Can you work these out from the model? Positions are in its coordinate system, mm. A direction names the side the tool comes from. Coordinates: 2 decimals unless noted, no trailing zeros. Loops run counter-clockwise (first coordinate to the right, second up) from the corner with the lowest first, then second, coordinate; pieces in that order, holes last.
```python
from build123d import *

# Parameters (mm, degrees)
SKETCH1_W           = 34.0614
SKETCH1_H           = 60
BOSS_EXTRUDE1_DEPTH = 8.9916
SKETCH2_W           = 34.0614
SKETCH2_H           = 8.9916
BOSS_EXTRUDE2_DEPTH = 51.0084
CUT_EXTRUDE2_REACH  = 10.992
SKETCH5_R           = 2.7686
SKETCH5_R_2         = 2.6416
CUT_EXTRUDE3_REACH  = 62
SKETCH6_R           = 2.7686
BOSS_EXTRUDE3_DEPTH = 34.0614
FILLET1_R           = 4.4958


with BuildPart() as part:
    # Sketch1 → Boss-Extrude1 (new body)
    with BuildSketch(Plane(origin=(0, 0, 0), x_dir=(0, 0, -1), z_dir=(1, 0, 0))):
        Rectangle(SKETCH1_W, SKETCH1_H)
    extrude(amount=BOSS_EXTRUDE1_DEPTH)

    # Sketch2 → Boss-Extrude2 (add)
    with BuildSketch(Plane(origin=(8.9916, 0, 0), x_dir=(0, 0, -1), z_dir=(1, 0, 0))):
        with Locations((0, 25.5042)):
            Rectangle(SKETCH2_W, SKETCH2_H)
    extrude(amount=BOSS_EXTRUDE2_DEPTH)

    # Sketch5 → Cut-Extrude2 (cut, up to next)
    with BuildSketch(Plane(origin=(8.9916, 0, 0), x_dir=(0, 0, -1), z_dir=(1, 0, 0)), mode=Mode.PRIVATE) as cut_extrude2_sk1:
        with Locations((-10.0076, -4.4958)):
            Circle(SKETCH5_R)
    cut_extrude2_tool1 = extrude(cut_extrude2_sk1.sketch, amount=-CUT_EXTRUDE2_REACH, mode=Mode.PRIVATE) & part.part
    add(cut_extrude2_tool1.solids().sort_by_distance((8.9916, -4.4958, 10.0076))[0], mode=Mode.SUBTRACT)
    # Sketch5 → Cut-Extrude2 (cut, up to next)
    with BuildSketch(Plane(origin=(8.9916, 0, 0), x_dir=(0, 0, -1), z_dir=(1, 0, 0)), mode=Mode.PRIVATE) as cut_extrude2_sk2:
        with Locations((10.0076, -4.4958)):
            Circle(SKETCH5_R_2)
    cut_extrude2_tool2 = extrude(cut_extrude2_sk2.sketch, amount=-CUT_EXTRUDE2_REACH, mode=Mode.PRIVATE) & part.part
    add(cut_extrude2_tool2.solids().sort_by_distance((8.9916, -4.4958, -10.0076))[0], mode=Mode.SUBTRACT)

    # Sketch6 → Cut-Extrude3 (cut, up to next)
    with BuildSketch(Plane(origin=(0, 30, 0), x_dir=(1, 0, 0), z_dir=(0, 1, 0)), mode=Mode.PRIVATE) as cut_extrude3_sk1:
        with Locations((41.995718, 10.0076)):
            Circle(SKETCH6_R)
    cut_extrude3_tool1 = extrude(cut_extrude3_sk1.sketch, amount=-CUT_EXTRUDE3_REACH, mode=Mode.PRIVATE) & part.part
    add(cut_extrude3_tool1.solids().sort_by_distance((41.995718, 30, -10.0076))[0], mode=Mode.SUBTRACT)
    # Sketch6 → Cut-Extrude3 (cut, up to next)
    with BuildSketch(Plane(origin=(0, 30, 0), x_dir=(1, 0, 0), z_dir=(0, 1, 0)), mode=Mode.PRIVATE) as cut_extrude3_sk2:
        with Locations((41.995718, -10.0076)):
            Circle(SKETCH6_R)
    cut_extrude3_tool2 = extrude(cut_extrude3_sk2.sketch, amount=-CUT_EXTRUDE3_REACH, mode=Mode.PRIVATE) & part.part
    add(cut_extrude3_tool2.solids().sort_by_distance((41.995718, 30, 10.0076))[0], mode=Mode.SUBTRACT)

    # Sketch7 → Boss-Extrude3 (add)
    with BuildSketch(Plane.XY.offset(17.0307)):
        Polygon((8.9916, 21.0084), (8.9916, 5.37450259), (24.62549741, 21.0084), align=None)
    extrude(amount=-BOSS_EXTRUDE3_DEPTH)

    # Fillet1
    fillet1_edges = [part.edges().sort_by_distance(p)[0] for p in [
        (8.9916, -30, 0),
        (60, 21.0084, 0),
    ]]
    fillet(fillet1_edges, radius=FILLET1_R)


solid = part.part
```
(1) I'm going to push flat-ended pins straight in: pin 1 (9 mm diameter, centred on x = 42, z = -10.01, fed in from -Y); pin 2 (3.5 mm diameter, centred on y = -4.5, z = 10.01, fed in from +X); pin 3 (8.5 mm diameter, centred on y = -4.5, z = -10.01, fed in from +X); pin 4 (6 mm diameter, centred on y = 3, z = -9, fed in from +X). Where does each tip first touch, or does it pass through?
Check values:
pin 1: stops at y = 21.01
pin 2: passes through
pin 3: stops at x = 8.99
pin 4: stops at x = 9.62
(2) I want a section at C-C on z = 9. Write out the boundary of the cut face in (x, y), then the cut area to 3 significant figures.
Check values:
outline: (0, -30) - (4.5, -30) arc R4.5 ccw to (8.99, -25.5) - (8.99, -7.07) - (0, -7.07) - close; (0, -1.92) - (8.99, -1.92) - (8.99, 5.37) - (24.63, 21.01) - (39.42, 21.01) - (39.42, 30) - (0, 30) - close; (44.57, 21.01) - (55.5, 21.01) arc R4.5 ccw to (60, 25.5) - (60, 30) - (44.57, 30) - close
area: 1,020 mm2
(3) If we mould it in two halves opening along X, with no side actions, what happens to faces 3 (the flat face through (60, 28, 0)), 4 (the cylindrical face through (4.56, -6.1, -7.91)), 5 (the cylindrical face through (43.273, 25.567, 12.464)), 6 (the flat face through (0, 0, 0))? For each: released by +X, released by -X, zero draft, split by the parting line, or undercut.
Check values:
face 3: released by +X
face 4: zero draft
face 5: undercut
face 6: released by -X
(4) I want a section at B-B on x = 41. Write out the boundary of the cut face in (y, z), then the cut area to 3 significant figures.
Check values:
outline: (21.01, -17.03) - (30, -17.03) - (30, -12.59) - (21.01, -12.59) - close; (21.01, -7.42) - (30, -7.42) - (30, 7.42) - (21.01, 7.42) - close; (21.01, 12.59) - (30, 12.59) - (30, 17.03) - (21.01, 17.03) - close
area: 213 mm2
(5) I want a section at D-D on x = 7. Write out the boundary of the cut face in (y, z).
Check values:
outline: (-29.24, -17.03) - (30, -17.03) - (30, 17.03) - (-29.24, 17.03) - close; hole circle Ø5.54 at (-4.5, 10.01); hole circle Ø5.28 at (-4.5, -10.01)
(6) I want a section at A-A on z = 2. Write out the boundary of the cut face in (x, y), then the cut area to 3 significant figures.
Check values:
outline: (0, -30) - (4.5, -30) arc R4.5 ccw to (8.99, -25.5) - (8.99, 5.37) - (24.63, 21.01) - (55.5, 21.01) arc R4.5 ccw to (60, 25.5) - (60, 30) - (0, 30) - close
area: 1,110 mm2
(7) Which directions (+Z, -Z, +X, -X, +Y, -Y) give clear straight access to the entire face, cutting with the end or side of a thin tool? Please do faces 1 (the cylindrical face through (44.636, 25.567, -10.839)), 2 (the flat face through (40, 21.008, 0)).
Check values:
face 1: +Y, -Y
face 2: +Z, -Z, +X, -Y
(8) If I drill on probe 1 along X at (y, z) = (-1.5, 4.5); probe 2 along Y at (x, z) = (49, 5); probe 3 along Y at (x, z) = (19, 3.5), over which ranges is the centre line in solid material (lowest first)?
Check values:
probe 1: x = 0 to 8.99
probe 2: y = 21.01 to 30
probe 3: y = 15.38 to 30
